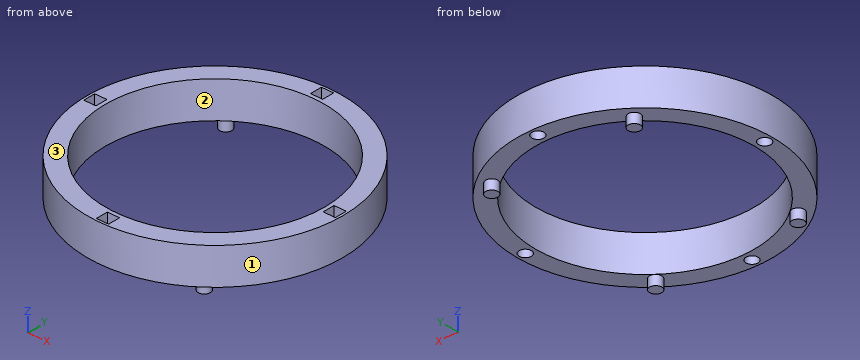
from build123d import *

# Parameters (mm, degrees)
SKETCH_R        = 52.5
SKETCH_R_2      = 45
PAD_DEPTH       = 15
SKETCH001_W     = 5
SKETCH001_H     = 5
POCKET001_DEPTH = 7
SKETCH002_R     = 2.5
HOLE_DEPTH      = 15.001
SKETCH012_R     = 2.495
PAD005_DEPTH    = 4


with BuildPart() as part:
    # Sketch → Pad (new body)
    with BuildSketch(Plane.XY):
        with Locations((52.5, 52.5)):
            Circle(SKETCH_R)
        with Locations((52.5, 52.5)):
            Circle(SKETCH_R_2, mode=Mode.SUBTRACT)
    extrude(amount=PAD_DEPTH)

    # Sketch001 (on Face4 of Pad) → Pocket001 (cut)
    with BuildSketch(Plane.XY.offset(15)):
        with Locations((3.5, 52.5)):
            Rectangle(SKETCH001_W, SKETCH001_H)
        with Locations((52.5, 3.5)):
            Rectangle(SKETCH001_W, SKETCH001_H)
        with Locations((101.5, 52.5)):
            Rectangle(SKETCH001_W, SKETCH001_H)
        with Locations((52.5, 101.5)):
            Rectangle(SKETCH001_W, SKETCH001_H)
    extrude(amount=-POCKET001_DEPTH, mode=Mode.SUBTRACT)

    # Sketch002 (on Face3 of Pocket001) → Hole (cut, through all)
    with BuildSketch(Plane.XY.offset(15)):
        with Locations((52.5, 101.5)):
            Circle(SKETCH002_R)
        with Locations((52.5, 3.5)):
            Circle(SKETCH002_R)
        with Locations((3.5, 52.5)):
            Circle(SKETCH002_R)
        with Locations((101.5, 52.5)):
            Circle(SKETCH002_R)
    extrude(amount=-HOLE_DEPTH, mode=Mode.SUBTRACT)

    # Sketch012 → Pad005 (join)
    with BuildSketch(Plane.XY):
        with Locations((81.6629049479, 90)):
            Circle(SKETCH012_R)
        with Locations((81.6629049479, 15)):
            Circle(SKETCH012_R)
        with Locations((23.3370950521, 90)):
            Circle(SKETCH012_R)
        with Locations((23.3370950521, 15)):
            Circle(SKETCH012_R)
    extrude(amount=-PAD005_DEPTH)


solid = part.part
Work out the finished part from the listing and answer in its coordinate system (mm). Face numbers are marked on the shaded views. Round coordinates to 2 decimals unless told otherwise and drop trailing zeros. Loops run counter-clockwise (first coordinate to the right, second up) from the corner with the lowest first, then second, coordinate; pieces in that order, holes last. Notation, with made-up numbers: (-12.75, -39.75) -> (-1.75, -39.75) arc R19 cw to (-1.75, -13.75) -> close; hole circle Ø2 at (54, 12). An arc over 180 degrees is marked (long way). Use one line per item in the form item = value.
(1) Find section B-B on x = 29. Give the vertices of the cut face in (y, z), then the cut area to 3 significant figures.
Answer list:
outline = (5.55, 0) -> (14.12, 0) -> (14.12, 15) -> (5.55, 15) -> close; (90.88, 0) -> (99.45, 0) -> (99.45, 15) -> (90.88, 15) -> close
area = 257 mm2
(2) Find section A-A on y = 73.5. Give the vertices of the cut face in (x, z).
Answer list:
outline = (4.38, 0) -> (12.7, 0) -> (12.7, 15) -> (4.38, 15) -> close; (92.3, 0) -> (100.62, 0) -> (100.62, 15) -> (92.3, 15) -> close
(3) Find section C-C on z = 9.25. Give the vertices of the cut face in (x, y).
Answer list:
outline = circle Ø105 at (52.5, 52.5); hole (1, 50) -> (6, 50) -> (6, 55) -> (1, 55) -> close; hole circle Ø90 at (52.5, 52.5); hole (50, 1) -> (55, 1) -> (55, 6) -> (50, 6) -> close; hole (50, 99) -> (55, 99) -> (55, 104) -> (50, 104) -> close; hole (99, 50) -> (104, 50) -> (104, 55) -> (99, 55) -> close
(4) Find section D-D on y = 15. Give the vertices of the cut face in (x, z).
Answer list:
outline = (15.76, 0) -> (20.84, 0) -> (20.84, -4) -> (25.83, -4) -> (25.83, 0) -> (27.63, 0) -> (27.63, 15) -> (15.76, 15) -> close; (77.37, 0) -> (79.17, 0) -> (79.17, -4) -> (84.16, -4) -> (84.16, 0) -> (89.24, 0) -> (89.24, 15) -> (77.37, 15) -> close
(5) For a pull along Y with two mould halves and no side action, classify the marked faces 1, 2 and 3 as released by +Y, released by -Y, zero draft, split by the parting line, or undercut.
Answer list:
face_1 = split by the parting line
face_2 = undercut
face_3 = zero draft
(6) Flat-ended cylindrical pins translate along their axes: P1, Ø2.5, axis at y = 53, z = 11, coming from the -X side; P2, Ø4, axis at y = 4, z = 13, coming from the -X side; P3, Ø10, axis at x = 91.5, z = 11, coming from the -Y side; P4, Ø1.5, axis at x = 51.5, z = 11, coming from the +Y side. Find the tip coordinate at first contact, or state that the pin passes through.
Answer list:
P1 = 0
P2 = 28.13
P3 = 12.5
P4 = 105
(7) Straight lines are drawn through the part: line 1 (Y direction, x = 52.5, z = 11.5); line 2 (X direction, y = 28.5, z = 9.75); line 3 (X direction, y = 43, z = 13). For each, find the intervals that lie inside material, in ascending order.
Answer list:
line_1 = 0 to 1, 6 to 7.5, 97.5 to 99, 104 to 105
line_2 = 5.81 to 14.43, 90.57 to 99.19
line_3 = 0.87 to 8.51, 96.49 to 104.13
